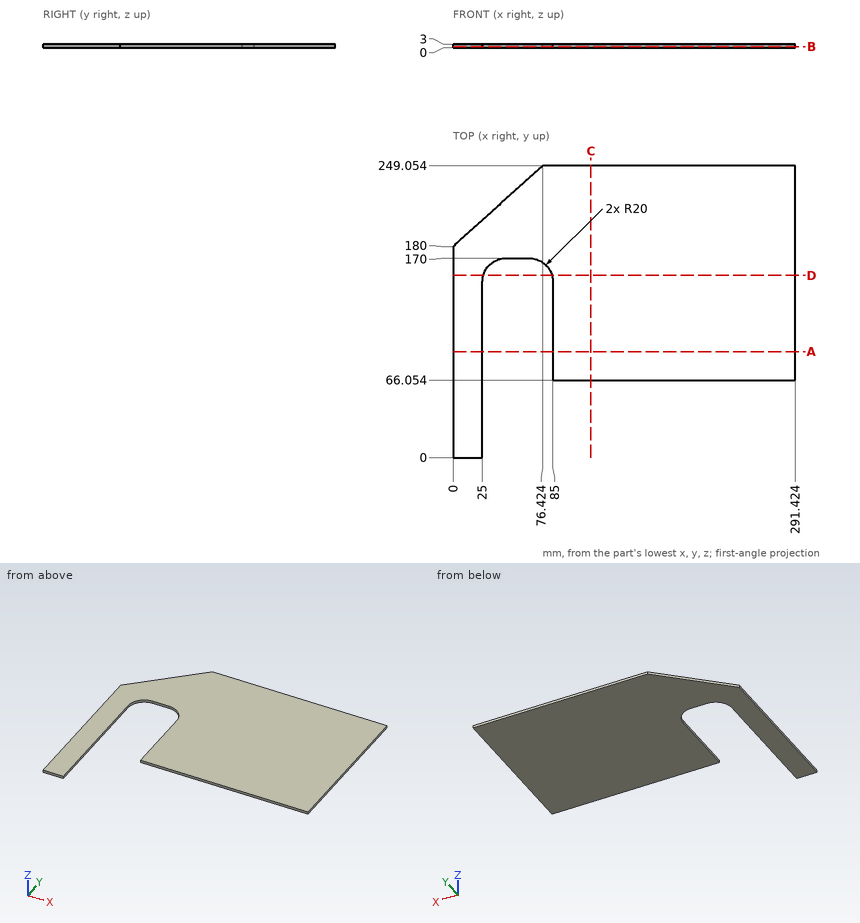
Answer from the drawing. Dimensions are ordinates in mm from the lowest x, y and z of the part. Give positions to 0.01 mm unless a question says otherwise; leave off trailing zeros. Write each loop counter-clockwise with the first axis right and the second up, starting at its lowest first coordinate (ties: lowest second). Pieces come first, ordered by that corner, then holes.
1) Given P1, Ø0.9, axis at y = 126.5, z = 2, coming from the -X side; P2, Ø1.5, axis at x = 173.5, z = 2, coming from the -Y side; P3, Ø0.9, axis at x = 53.5, z = 1.5, coming from the -Y side, each flat-ended and moving along its own axis, determine where each tip first touches the part or whether it passes through.
2) Section D-D (y = 155.5) is taken. Write down the section's boundary in (x, z).
3) Section C-C (x = 117.5) is taken. Write down the section's boundary in (y, z).
4) Find the intervals of material crossed by L1, parallel to X at y = 121.5, z = 0.7; L2, parallel to X at y = 35, z = 2.45; L3, parallel to Y at x = 163, z = 1.85, in increasing order.
5) Section A-A (y = 90.5) is taken. Write down the section's boundary in (x, z).
6) Section B-B (z = 0.85) is taken. Write down the section's boundary in (x, y).
Response:
1. P1: stops at x = 0
1. P2: stops at y = 66.05
1. P3: stops at y = 170
2. outline: (0, 0) - (25.77, 0) - (25.77, 3) - (0, 3) - close; (84.23, 0) - (291.42, 0) - (291.42, 3) - (84.23, 3) - close
3. outline: (66.05, 0) - (249.05, 0) - (249.05, 3) - (66.05, 3) - close
4. L1: x = 0 to 25, 85 to 291.42
4. L2: x = 0 to 25
4. L3: y = 66.05 to 249.05
5. outline: (0, 0) - (25, 0) - (25, 3) - (0, 3) - close; (85, 0) - (291.42, 0) - (291.42, 3) - (85, 3) - close
6. outline: (0, 0) - (25, 0) - (25, 150) arc R20 cw to (45, 170) - (65, 170) arc R20 cw to (85, 150) - (85, 66.05) - (291.42, 66.05) - (291.42, 249.05) - (76.42, 249.05) - (0, 180) - close
